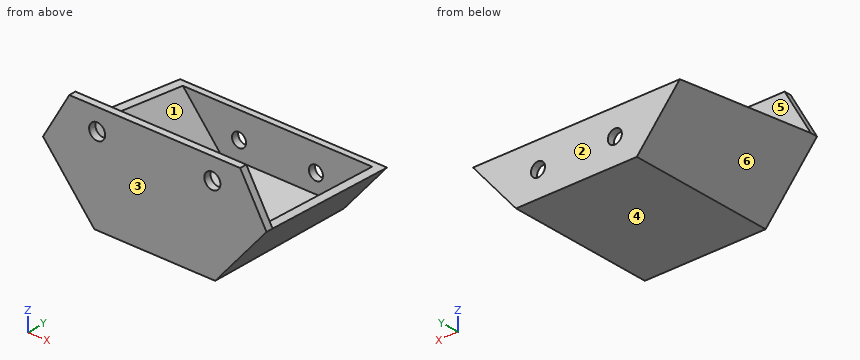
```python
from build123d import *

# Parameters (mm, degrees)
EXTRUDE_1_DEPTH          = 211
SHELL_1_T                = 10
CUT_EXTRUDE_1_DEPTH      = 306.363666708
CUT_EXTRUDE_1_DEPTH_BACK = 306.363666708
CUT_EXTRUDE_2_DEPTH      = 306.363666708
CUT_EXTRUDE_2_DEPTH_BACK = 40
SKETCH_3_R               = 10
SKETCH_4_R               = 11.451002367
CUT_EXTRUDE_3_DEPTH      = 40


with BuildPart() as part:
    # 草图1 → 凸台-拉伸1 (new body)
    with BuildSketch(Plane(origin=(0, 0, 0), x_dir=(1, 0, 0), z_dir=(0, 1, 0))):
        Polygon((122, 0), (-122, 0), (-159.592352403, 65.111864338), (-86.265, 152.5), (86.265, 152.5), (159.592352403, 65.111864338), align=None)
    extrude(amount=EXTRUDE_1_DEPTH)

    # 抽壳1 (no face opened: a closed hollow body)
    add(offset(amount=-SHELL_1_T, mode=Mode.PRIVATE), mode=Mode.SUBTRACT)

    # 草图2 → 切除-拉伸1 (cut, two sides: drawn at the far end of the back side and taken through both)
    with BuildSketch(Plane(origin=(0, 0, 0), x_dir=(0, 0, -1), z_dir=(1, 0, 0)).offset(-CUT_EXTRUDE_1_DEPTH_BACK)):
        Polygon((79.3, 211), (65.111864338, 10), (0, 10), (0, 211), align=None)
    extrude(amount=CUT_EXTRUDE_1_DEPTH + CUT_EXTRUDE_1_DEPTH_BACK, mode=Mode.SUBTRACT)

    # 草图3 → 切除-拉伸2 (cut, two sides: drawn at the far end of the back side and taken through both)
    with BuildSketch(Plane(origin=(0, 211, 0), x_dir=(1, 0, 0), z_dir=(0, 1, 0)).offset(-CUT_EXTRUDE_2_DEPTH_BACK)):
        with Locations(Location((-54.9, 115.9, 0), (0, 0, 90))):
            Circle(SKETCH_3_R)
        with Locations(Location((54.9, 115.9, 0), (0, 0, 90))):
            Circle(SKETCH_3_R)
    extrude(amount=CUT_EXTRUDE_2_DEPTH + CUT_EXTRUDE_2_DEPTH_BACK, mode=Mode.SUBTRACT)

    # 草图4 → 切除-拉伸3 (cut)
    with BuildSketch(Plane(origin=(0, 10, 0), x_dir=(1, 0, 0), z_dir=(0, 1, 0))):
        with Locations(Location((-82.25, 30.5, 0), (0, 0, 270))):
            Circle(SKETCH_4_R)
        with Locations(Location((82.25, 30.5, 0), (0, 0, 270))):
            Circle(SKETCH_4_R)
    extrude(amount=-CUT_EXTRUDE_3_DEPTH, mode=Mode.SUBTRACT)


solid = part.part
```
Part model, mm, in its own coordinate system. Face numbers are marked on the shaded views. A direction names the side the tool comes from. Give positions to 0.01 mm unless a question says otherwise; leave off trailing zeros. Write each loop counter-clockwise with the first axis right and the second up, starting at its lowest first coordinate (ties: lowest second). Pieces come first, ordered by that corner, then holes. Notation, with made-up numbers: M 50.25,-15 L 67.25,-15 A9 ccw 67.25,-5 Z; hole C 37,42.25 d2. An arc over 180 degrees is marked long. Use CSV: the item, a comma, the result in double quotes.
Item 1: Slice it at A-A on x = -54.9. Write the cut outline in (y, z), plus the area to 3 significant figures.
Taken from the geometry:
outline,"M 0,-152.5 L 211,-152.5 L 211,-125.9 L 201,-125.9 L 201,-142.5 L 10,-142.5 L 10,0 L 0,0 Z; M 201,-105.9 L 211,-105.9 L 211,-79.3 L 201,-78.59 Z"
area,"3,970 mm²"
Item 2: Which spindle directions (+Z, -Z, +X, -X, +Y, -Y) get a long thin tool onto all of the face, cutting with end or side? Do the marked faces 5 and 6. Say none if no direction does.
Taken from the geometry:
face 5,"+Z"
face 6,"-Z, -X, +Y, -Y"
Item 3: Pull direction Y, two halves, no side cores. Call the marked faces 1, 2, 3 and 4: +Y half, -Y half, draft (parallel to the pull), parting line (faces both ways), or undercut.
Taken from the geometry:
face 1,"undercut"
face 2,"+Y half"
face 3,"-Y half"
face 4,"draft"
Item 4: Drill centre lines: probe 1 along Y at (x, z) = (-8, -105); probe 2 along X at (y, z) = (208, -115.9); probe 3 along Z at (x, y) = (82, 6). Where is each one in solid material? Low to high.
Taken from the geometry:
probe 1,"y = 0 to 10, 201 to 211"
probe 2,"x = -116.98 to -64.9, -44.9 to 44.9, 64.9 to 116.98"
probe 3,"z = -152.5 to -41.95, -19.05 to 0"
Item 5: Slice it at B-B on z = -109.5. Write the cut outline in (x, y), plus the area to 3 significant figures.
Taken from the geometry:
outline,"M -122.35,0 L 122.35,0 L 122.35,211 L 62.58,211 L 62.58,201 L 109.29,201 L 109.29,10 L -109.29,10 L -109.29,201 L -62.58,201 L -62.58,211 L -122.35,211 Z; M -47.22,201 L 47.22,201 L 47.22,211 L -47.22,211 Z"
area,"9,570 mm²"
Item 6: Slice it at C-C on y = 115.5. Write the cut outline in (x, z) (1 decimal), plus the area to 3 significant figures.
Taken from the geometry:
outline,"M -153.3,-72.6 L -86.3,-152.5 L 86.3,-152.5 L 153.3,-72.6 L 140.3,-72.6 L 81.6,-142.5 L -81.6,-142.5 L -140.3,-72.6 Z"
area,"3,640 mm²"
Item 7: Pin check, flat tips, straight feed: P1, Ø2, axis at x = 63.5, y = 126.5, coming from the +Z side; P2, Ø10, axis at x = -62, z = -65, coming from the +Y side; P3, Ø1.5, axis at x = -46.5, z = -81, coming from the -Y side; P4, Ø12, axis at y = 39.5, z = -125, coming from the +X side. Stop position of each tip, or through.
Taken from the geometry:
P1,"stops at z = -142.5"
P2,"stops at y = 10"
P3,"stops at y = 0"
P4,"stops at x = 114.37"
Item 8: Slice it at D-D on z = -30.5. Write the cut outline in (x, y).
Taken from the geometry:
outline,"M -139.61,0 L -93.7,0 L -93.7,10 L -139.61,10 Z; M -70.8,0 L 70.8,0 L 70.8,10 L -70.8,10 Z; M 93.7,0 L 139.61,0 L 139.61,10 L 93.7,10 Z"
